Input: part model. Units: mm. Frame: model coordinates. A direction names the side the tool comes from. Coordinates: 2 decimals unless noted, no trailing zeros. Write each loop counter-clockwise with the first axis right and the second up, starting at its lowest first coordinate (ties: lowest second). Pieces come first, ordered by that corner, then holes. Notation, with made-up numbers: M -21,30 L -6,30 A19 ccw -6,62 Z; hole C 76,15 d7. An arc over 180 degrees is marked long. Answer as a JSON object with one key per item and string values. Group by question number.
from build123d import *

# Parameters (mm, degrees)
F1_DEPTH = 3.81
F2_W     = 6.1722
F2_H     = 37.9222
F3_DEPTH = 3.811


with BuildPart() as f1:
    # F0 (on Top) → F1 (new body)
    with BuildSketch(Plane.XY):
        Polygon((25.4889, 127), (0, 127), (0, 101.5111), (6.2611, 101.5111), (6.2611, 76.2889), (0, 76.2889), (0, 50.7111), (6.2611, 50.7111), (6.2611, 25.4889), (0, 25.4889), (0, 0), (25.4889, 0), (25.4889, 6.2611), (50.7111, 6.2611), (50.7111, 0), (76.2889, 0), (76.2889, 6.2611), (101.5111, 6.2611), (101.5111, 0), (127.0889, 0), (127.0889, 6.2611), (152.3111, 6.2611), (152.3111, 0), (177.8, 0), (177.8, 25.4889), (171.5389, 25.4889), (171.5389, 50.7111), (177.8, 50.7111), (177.8, 76.2889), (171.5389, 76.2889), (171.5389, 101.5111), (177.8, 101.5111), (177.8, 127), (152.3111, 127), (152.3111, 120.7389), (127.0889, 120.7389), (127.0889, 127), (101.5111, 127), (101.5111, 120.7389), (76.2889, 120.7389), (76.2889, 127), (50.7111, 127), (50.7111, 120.7389), (25.4889, 120.7389), align=None)
    extrude(amount=F1_DEPTH)

    # F2 (on face) → F3 (cut, through all)
    with BuildSketch(Plane.XY.offset(3.81)):
        with Locations((88.9, 88.9)):
            Rectangle(F2_W, F2_H)
        with Locations((88.9, 38.1)):
            Rectangle(F2_W, F2_H)
    extrude(amount=-F3_DEPTH, mode=Mode.SUBTRACT)


solid = f1.part
Q1. Draft query along X for faces 4 (the flat face through (3, 101.511, 2)), 5 (the flat face through (152.311, 3, 2)), 6 (the flat face through (171.539, 38, 2)). Return one class per face: released by +X, released by -X, zero draft, split by the parting line, or undercut.
Q2. Section C-C, the plane y = 55. Return the cut outline in (x, z).
Q3. Line query: line 1 (X direction, y = 45, z = 3.05); line 2 (X direction, y = 52, z = 2); line 3 (Y direction, x = 97, z = 2.5). Output: solid intervals per line, ascending. Write a range as from..to.
Q4. Access query for faces 1 (the flat face through (171.539, 89, 2)), 2 (the flat face through (89, 19.139, 2)), 3 (the flat face through (101.511, 3, 2)). Directions: +Z, -Z, +X, -X, +Y, -Y. A direction counts if a zero-diameter tool reaches every point of the face in a straight line with its end or side. Return the directions, or none.
Q5. Pin query (flat end, axial travel): pin 1 Ø1.1 at (x, z) = (90.5, 2) entering from -Y; pin 2 Ø1.9 at (y, z) = (40, 1.5) entering from -X; pin 3 Ø1.5 at (y, z) = (101, 1.5) entering from -X; pin 4 Ø1.1 at (x, z) = (88, 1.5) entering from +Y. Return the tip coordinate at first contact, or that it passes through.
Q6. Section D-D, the plane x = 32. Return the cut outline in (y, z).
Q7. Section A-A, the plane y = 38. Return the cut outline in (x, z).
Q8. Section B-B, the plane z = 1.65. State how many separate pieces and enclosed holes the cut face has, and give its area (3 significant figures).
Filled in:
{
 "1": {"face 4": "zero draft", "face 5": "undercut", "face 6": "released by +X"},
 "2": {"outline": "M 0,0 L 85.81,0 L 85.81,3.81 L 0,3.81 Z; M 91.99,0 L 177.8,0 L 177.8,3.81 L 91.99,3.81 Z"},
 "3": {"line 1": "6.26..85.81, 91.99..171.54", "line 2": "0..85.81, 91.99..177.8", "line 3": "6.26..120.74"},
 "4": {"face 1": "+Z, -Z, +X", "face 2": "+Z, -Z", "face 3": "+Z, -Z, -Y"},
 "5": {"pin 1": "y = 6.26", "pin 2": "x = 6.26", "pin 3": "x = 0", "pin 4": "y = 120.74"},
 "6": {"outline": "M 6.26,0 L 120.74,0 L 120.74,3.81 L 6.26,3.81 Z"},
 "7": {"outline": "M 6.26,0 L 85.81,0 L 85.81,3.81 L 6.26,3.81 Z; M 91.99,0 L 171.54,0 L 171.54,3.81 L 91.99,3.81 Z"},
 "8": {"separate pieces": "1", "enclosed holes": "2", "area": "20,500 mm^2"}
}
